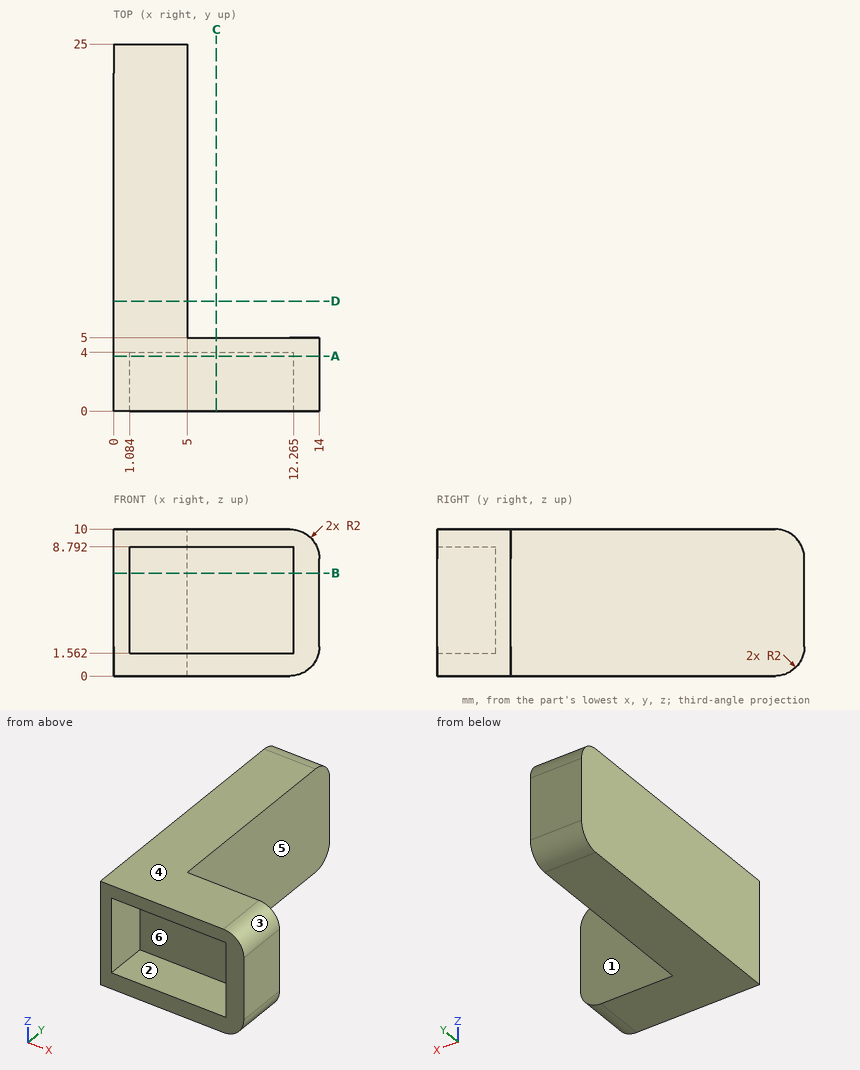
Part print with two shaded views. Sizes in mm from the minimum x, y, z corner. A direction names the side the tool comes from. Round coordinates to 2 decimals unless told otherwise and drop trailing zeros. Loops run counter-clockwise (first coordinate to the right, second up) from the corner with the lowest first, then second, coordinate; pieces in that order, holes last. Notation, with made-up numbers: (85, 63) - (116, 63) arc R21 ccw to (116, 98) - close; hole circle Ø7 at (33.25, 56.25). An arc over 180 degrees is marked (long way). Put each result on its own line as item: value.
1. Slice it at D-D on y = 7.5. List the corners of the cut face in (x, z), and give its area (3 significant figures).
Geometry check:
outline: (0, 0) - (5, 0) - (5, 10) - (0, 10) - close
area: 50.0 mm²
2. Slice it at C-C on x = 7. List the corners of the cut face in (y, z).
Geometry check:
outline: (0, 0) - (5, 0) - (5, 10) - (0, 10) - (0, 8.79) - (4, 8.79) - (4, 1.56) - (0, 1.56) - close
3. Wall check: line 1 (X direction, y = 14, z = 5.5); line 2 (Y direction, x = 4.5, z = 4.25); line 3 (Z direction, x = 9.25, y = 3.25). Give the ranges that are in metal, low to high.
Geometry check:
line 1: 0 to 5
line 2: 4 to 25
line 3: 0 to 1.56, 8.79 to 10
4. Pin check, flat tips, straight feed: P1, Ø1.2, axis at y = 3, z = 7, coming from the -X side; P2, Ø1, axis at y = 7.5, z = 5.5, coming from the +X side; P3, Ø4.5, axis at x = 11, z = 7.5, coming from the +Y side. Stop position of each tip, or through.
Geometry check:
P1: x = 0
P2: x = 5
P3: y = 5
5. 3-axis set-ups, long thin cutter, end or side, ignore diameter. For the marked faces 4, 5 and 6: which of +Z, -Z, +X, -X, +Y, -Y reach the whole face in a straight line?
Geometry check:
face 4: +Z, +X, -X, +Y, -Y
face 5: +Z, -Z, +X, +Y
face 6: -Y
6. Two-plate mould, pull along Z, no slides. Class the marked faces 1, 2 and 3: released by +Z, released by -Z, zero draft, split by the parting line, or undercut.
Geometry check:
face 1: zero draft
face 2: undercut
face 3: released by +Z
7. Slice it at B-B on z = 7. List the corners of the cut face in (x, y) (1 decimal), and give its area (3 significant figures).
Geometry check:
outline: (0, 0) - (1.1, 0) - (1.1, 4) - (12.3, 4) - (12.3, 0) - (14, 0) - (14, 5) - (5, 5) - (5, 25) - (0, 25) - close
area: 125 mm²
8. Slice it at A-A on y = 3.75. List the corners of the cut face in (x, z) (1 decimal).
Geometry check:
outline: (0, 0) - (12, 0) arc R2 ccw to (14, 2) - (14, 8) arc R2 ccw to (12, 10) - (0, 10) - close; hole (1.1, 1.6) - (12.3, 1.6) - (12.3, 8.8) - (1.1, 8.8) - close
